from build123d import *

# Parameters (mm, degrees)
F1_DEPTH = 2
F2_R     = 8.5
F3_DEPTH = 2
F4_SIZE  = 1.99999
F6_DEPTH = 4
F7_R     = 4
F8_DEPTH = 8


# Not quite as in the source:
# - a fillet or chamfer is up to 0.001 mm smaller than in the source, because OpenCascade refuses the exact size


with BuildPart() as f1:
    # F0 (on Top) → F1 (new body)
    with BuildSketch(Plane.XY):
        with BuildLine():
            ThreePointArc((15, 10), (13.5355339059, 13.5355339059), (10, 15))
            Line((10, 15), (-10, 15))
            ThreePointArc((-10, 15), (-13.5355339059, 13.5355339059), (-15, 10))
            Line((-15, 10), (-15, -10))
            ThreePointArc((-15, -10), (-13.5355339059, -13.5355339059), (-10, -15))
            Line((-10, -15), (10, -15))
            ThreePointArc((10, -15), (13.5355339059, -13.5355339059), (15, -10))
            Line((15, -10), (15, 10))
        make_face()
    extrude(amount=F1_DEPTH)

    # F2 (on face) → F3 (join)
    with BuildSketch(Plane.XY.offset(2)):
        Circle(F2_R)
    extrude(amount=F3_DEPTH)

    # F4 (size 2 in the source; OpenCascade refuses exactly that, so slightly less here)
    f4_edges = [f1.edges().sort_by_distance(p)[0] for p in [
        (-8.5, 0, 4),
    ]]
    chamfer(f4_edges, length=F4_SIZE)

    # F5 (on face) → F6 (join)
    with BuildSketch(Plane.XY.offset(4)):
        Polygon((6.3508529611, 0), (3.1754264805, 5.5), (-3.1754264805, 5.5), (-6.3508529611, 0), (-3.1754264805, -5.5), (3.1754264805, -5.5), align=None)
    extrude(amount=F6_DEPTH)

    # F7 (on face) → F8 (join)
    with BuildSketch(Plane.XY.offset(8)):
        Circle(F7_R)
    extrude(amount=F8_DEPTH)


solid = f1.part
Build history of the part. All positions in model axes, mm. A direction names the side the tool comes from. Coordinates: 2 decimals unless noted, no trailing zeros. Order: outer loops, then holes, each group sorted by start corner. A loop starts at its lowest first (then second) coordinate and runs counter-clockwise, first axis right, second up. Notation, with made-up numbers: (-5, 20) - (35, 20) arc R18 ccw to (35, 45) - close; hole circle Ø4 at (-17, -17.75). An arc over 180 degrees is marked (long way). Put each result on its own line as item: value.
1. Saw through at B-B (z = 5.5). Write the cut outline in (x, y).
Answer sheet:
outline: (-6.35, 0) - (-3.18, -5.5) - (3.18, -5.5) - (6.35, 0) - (3.18, 5.5) - (-3.18, 5.5) - close
2. Tool access for faces 1 (the face through (4.785, 2.712, 5.972)), 2 (the face through (-4.785, -2.712, 5.972)), 3 (the face through (0, -5.5, 6)), 4 (the face through (0, 5.5, 6)): list every direction of +Z, -Z, +X, -X, +Y, -Y with a clear straight run to the whole face (end or side of a thin tool).
Answer sheet:
face 1: +Z, +X, +Y
face 2: +Z, -X, -Y
face 3: +Z, +X, -X, -Y
face 4: +Z, +X, -X, +Y
3. Drop flat-ended pins along their axis: P1, Ø15, axis at x = 1.5, y = 4.5, coming from the +Z side; P2, Ø6, axis at x = -4.5, y = -6.5, coming from the +Z side; P3, Ø6, axis at x = -3.5, z = 6.5, coming from the -Y side; P4, Ø4.5, axis at x = 1.5, z = 7, coming from the +Y side. Give the stop position or say it passes through.
Answer sheet:
P1: stops at z = 16
P2: stops at z = 8
P3: stops at y = -6.35
P4: stops at y = 5.5
4. Saw through at D-D (z = 3). Write the cut outline in (x, y).
Answer sheet:
outline: circle Ø15 at (0, 0)
5. Saw through at C-C (y = 12.75). Write the cut outline in (x, z).
Answer sheet:
outline: (-14.18, 0) - (14.18, 0) - (14.18, 2) - (-14.18, 2) - close
6. Probe line 1 along Z through (x, y) = (0, -6.25); line 2 along Z through (x, y) = (3.25, -3.5); line 3 along Y through (x, z) = (-1, 7.5). List the from-to ranges inside material, lowest first. Write a range as [from, to].
Answer sheet:
line 1: z = [0, 4]
line 2: z = [0, 8]
line 3: y = [-5.5, 5.5]
